Build history of the part. All positions in model axes, mm. Round coordinates to 2 decimals unless told otherwise and drop trailing zeros. Loops run counter-clockwise (first coordinate to the right, second up) from the corner with the lowest first, then second, coordinate; pieces in that order, holes last. Notation, with made-up numbers: (0, 82) - (41, 82) arc R21 cw to (41, 94) - close; hole circle Ø10 at (14.5, 36.5). An arc over 180 degrees is marked (long way). Use one line per item in the form item = value. Start each with the question number.
Q1. Pin check, flat tips, straight feed: pin 1 (1 mm diameter, centred on x = 4.5, y = 4, fed in from -Z); pin 2 (1.5 mm diameter, centred on x = -11.5, y = 3.5, fed in from +Z); pin 3 (1.5 mm diameter, centred on y = 3.5, z = -12.5, fed in from +X). Stop position of each tip, or through.
Q2. Saw through at B-B (z = 0). Give the cut face in (x, y), then the cut area to 3 significant figures.
Q3. Drill centre lines: line 1 (Z direction, x = 0, y = 3); line 2 (X direction, y = 2.15, z = -12); line 3 (X direction, y = 0.55, z = 16). Where is each one in solid material? Low to high.
Q4. Saw through at C-C (y = 1). Give the cut face in (x, z).
Q5. Saw through at A-A (x = 0). Give the cut face in (y, z), then the cut area to 3 significant figures.
Q6. Mould opens along Z. For faces 1 (the face through (-0.434, 2.218, 7.273)), 2 (the face through (0, 0, 2)), 3 (the face through (0, 2, 1)), 4 (the face through (-8.282, 2.218, 20.736)) say: released by +Z, released by -Z, zero draft, split by the parting line, or undercut.
Q7. Saw through at D-D (x = 2.5). Give the cut face in (y, z), then the cut area to 3 significant figures.
```python
from build123d import *

# Parameters (mm, degrees)
SKETCH1_R           = 1
SKETCH1_R_2         = 4
SKETCH1_R_3         = 2
BOSS_EXTRUDE1_DEPTH = 4.5


with BuildPart() as part:
    # Sketch1 → Boss-Extrude1 (new body)
    with BuildSketch(Plane(origin=(0, 0, 0), x_dir=(1, 0, 0), z_dir=(0, 1, 0))):
        with BuildLine():
            ThreePointArc((-13.216577068, -12.398039355), (-14.355594067, -15.696551109), (-12.358546854, -18.55825374))
            Line((-12.358546854, -18.55825374), (-4.089079858, -22.975728551))
            ThreePointArc((-4.089079858, -22.975728551), (5.687833956, -21.875689807), (8.154517998, -12.351321125))
            ThreePointArc((8.154517998, -12.351321125), (6.724685531, -0.7813357), (7.419863607, 10.855919606))
            ThreePointArc((7.419863607, 10.855919606), (-0.324076795, 19.500551353), (-7.293531269, 10.220197086))
            ThreePointArc((-7.293531269, 10.220197086), (-7.006184901, 1.034726978), (-8.662387246, -8.004765421))
            ThreePointArc((-8.662387246, -8.004765421), (-10.314906991, -10.000536559), (-12.253567388, -11.719699089))
            ThreePointArc((-12.253567388, -11.719699089), (-12.729149831, -12.067276987), (-13.216577068, -12.398039355))
        make_face()
        with Locations((-10.546429397, -15.165988669)):
            Circle(SKETCH1_R, mode=Mode.SUBTRACT)
        with Locations((0, -15.321013501)):
            Circle(SKETCH1_R_2, mode=Mode.SUBTRACT)
        with Locations((0, -5.321013501)):
            Circle(SKETCH1_R_3, mode=Mode.SUBTRACT)
        Circle(SKETCH1_R, mode=Mode.SUBTRACT)
        with Locations((-3e-08, 12)):
            Circle(SKETCH1_R_2, mode=Mode.SUBTRACT)
    extrude(amount=BOSS_EXTRUDE1_DEPTH)


solid = part.part
```
Report:
q1.pin_1 = -18.35
q1.pin_2 = 19.42
q1.pin_3 = 7.51
q2.outline = (-7.1, 0) - (-1, 0) - (-1, 4.5) - (-7.1, 4.5) - close; (1, 0) - (6.7, 0) - (6.7, 4.5) - (1, 4.5) - close
q2.area = 53.1 mm²
q3.line_1 = -19.51 to -16, -8 to -1, 1 to 3.32, 7.32 to 11.32, 19.32 to 24
q3.line_2 = -7.51 to -4, 4 to 7.51
q3.line_3 = -14.3 to -11.1, -9.99 to -3.94, 3.94 to 8.65
q4.outline = (-13.22, 12.4) arc R16.87 cw to (-8.66, 8) arc R43.33 cw to (-7.29, -10.22) arc R7.51 ccw (long way) to (7.42, -10.86) arc R63.92 cw to (8.15, 12.35) arc R8.68 ccw to (-4.09, 22.98) - (-12.36, 18.56) arc R3.85 ccw to start; hole circle Ø2 at (-10.55, 15.17); hole circle Ø8 at (0, -12); hole circle Ø8 at (0, 15.32); hole circle Ø4 at (0, 5.32); hole circle Ø2 at (0, 0)
q5.outline = (0, -19.51) - (4.5, -19.51) - (4.5, -16) - (0, -16) - close; (0, -8) - (4.5, -8) - (4.5, -1) - (0, -1) - close; (0, 1) - (4.5, 1) - (4.5, 3.32) - (0, 3.32) - close; (0, 7.32) - (4.5, 7.32) - (4.5, 11.32) - (0, 11.32) - close; (0, 19.32) - (4.5, 19.32) - (4.5, 24) - (0, 24) - close
q5.area = 96.8 mm²
q6.face_1 = undercut
q6.face_2 = zero draft
q6.face_3 = undercut
q6.face_4 = released by +Z
q7.outline = (0, -19.08) - (4.5, -19.08) - (4.5, -15.12) - (0, -15.12) - close; (0, -8.88) - (4.5, -8.88) - (4.5, 12.2) - (0, 12.2) - close; (0, 18.44) - (4.5, 18.44) - (4.5, 23.63) - (0, 23.63) - close
q7.area = 136 mm²
